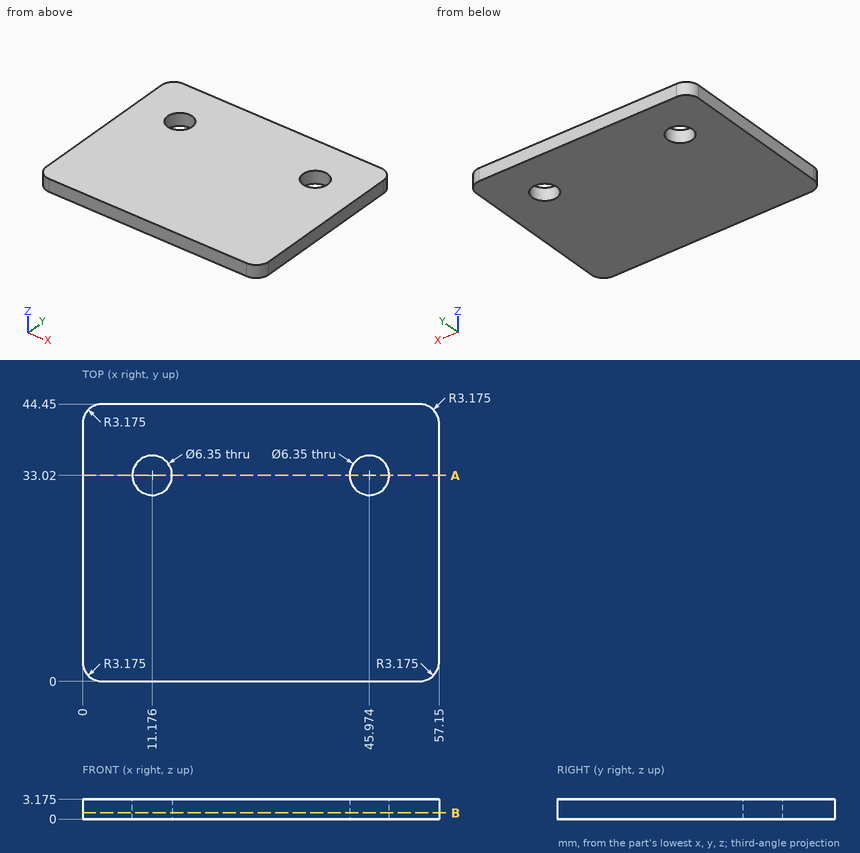
Could you check a few things on this drawing? It's one solid part, dimensions in mm from its lowest x, y, z. Coordinates: 2 decimals unless noted, no trailing zeros. Order: outer loops, then holes, each group sorted by start corner. A loop starts at its lowest first (then second) coordinate and runs counter-clockwise, first axis right, second up. Notation, with made-up numbers: M 26.25,11.25 L 31.25,11.25 A25 ccw 31.25,35.25 Z; hole C 65.25,52 d10. An arc over 180 degrees is marked long. Use a Markdown table: item, result. Add a question column.
Q1. If I drill on L1, parallel to Y at x = 11, z = 0.85; L2, parallel to X at y = 33, z = 1; L3, parallel to Y at x = 13, z = 1, over which ranges is the centre line in solid material (lowest first)?
Q2. I want a section at A-A on y = 33.02. List the corners of the cut face in (x, z) for me (3 decimals).
Q3. I want a section at B-B on z = 1. List the corners of the cut face in (x, y) for me (3 decimals), then the cut area to 3 significant figures.
Q4. I'm going to push a flat-ended pin straight in: pin 1 (5 mm diameter, centred on x = 45.974, y = 33.02, fed in from -Z). Where does the tip first touch, or does it pass through?
Checked values:
| question | item | result |
|---|---|---|
| 1 | L1 | 0 to 29.85, 36.19 to 44.45 |
| 1 | L2 | 0 to 8, 14.35 to 42.8, 49.15 to 57.15 |
| 1 | L3 | 0 to 30.42, 35.62 to 44.45 |
| 2 | outline | M 0,0 L 8.001,0 L 8.001,3.175 L 0,3.175 Z; M 14.351,0 L 42.799,0 L 42.799,3.175 L 14.351,3.175 Z; M 49.149,0 L 57.15,0 L 57.15,3.175 L 49.149,3.175 Z |
| 3 | outline | M 0,3.175 A3.175 ccw 3.175,0 L 53.975,0 A3.175 ccw 57.15,3.175 L 57.15,41.275 A3.175 ccw 53.975,44.45 L 3.175,44.45 A3.175 ccw 0,41.275 Z; hole C 11.176,33.02 d6.35; hole C 45.974,33.02 d6.35 |
| 3 | area | 2,470 mm² |
| 4 | pin 1 | through |
